Input: part model. Units: mm. Frame: model coordinates. Round coordinates to 2 decimals unless told otherwise and drop trailing zeros. Loops run counter-clockwise (first coordinate to the right, second up) from the corner with the lowest first, then second, coordinate; pieces in that order, holes last. Notation, with made-up numbers: (88, 72.5) -> (95, 72.5) arc R11 ccw to (95, 78.5) -> close; hole circle Ø8 at (60, 77). An arc over 180 degrees is marked (long way). Answer in a Markdown table with one row per item. Add a question column.
Q1. Pin query (flat end, axial travel): pin 1 (8 mm diameter, centred on y = 10.5, z = 4, fed in from +X); pin 2 (2 mm diameter, centred on y = -8.5, z = -0.5, fed in from -X). Return the tip coordinate at first contact, or that it passes through.
Q2. Section A-A, the plane z = -4.5. Output: boundary loops of the cut face in (x, y), and give its area (3 significant figures).
Q3. Mould query, pull axis X, two halves, no side actions, for faces 1 (the face through (13.404, -0.033, -6.511)), 2 (the face through (-13.404, -0.033, 6.511)), 3 (the face through (6.63, 0.87, 0.09)). Classes: pulls with the +X half, pulls with the -X half, needs draft (parallel to the pull), parting line crosses it, or undercut.
Q4. Ray query, L1, parallel to Y at x = 0, z = 2; L2, parallel to X at y = 2.75, z = 1.5; L3, parallel to Y at x = -2.25, z = -0.75. Return the intervals inside material, ascending. Write a range as from..to.
Solid Edge part; units mm, degrees
sketch "Sketch1" plane through (0, 0, 0) normal (0, 0, 1) x (1, 0, 0)
  line L0 (-7.5, -12.9904) -> (7.5, -12.9904)
  line L1 (7.5, -12.9904) -> (15, 0)
  line L2 (15, 0) -> (7.5, 12.9904)
  line L3 (7.5, 12.9904) -> (-7.5, 12.9904)
  line L4 (-7.5, 12.9904) -> (-15, 0)
  line L5 (-15, 0) -> (-7.5, -12.9904)
extrude "Protrusion1" add sketch "Sketch1" along normal mid plane 13.5
sketch "Sketch2" plane through (0, 0, 0) normal (1, 0, 0) x (0, 1, 0)
  line L0 (12.9904, -6.75) -> (34.5982, 5.7253)
revolve "RevolvedCutout1" cut sketch "Sketch2" angle 360 about axis through (0, 0, -57) along (0, 0, 1) material side at (0, 23.8193, -0.5557)
mirror "Mirror1" about plane through (0, 0, 0) normal (0, 0, 1) of "RevolvedCutout1"
hole "Hole_1" at (0, 0, 6.75) direction (0, 0, -1) diameter 13.376 end through all
properties part number "5" material "Fe - 410 W"
Answer block:
| question | item | result |
|---|---|---|
| 1 | pin 1 | x = 11.25 |
| 1 | pin 2 | x = -10.67 |
| 2 | outline | (-15, 0) -> (-7.5, -12.99) -> (7.5, -12.99) -> (15, 0) -> (7.5, 12.99) -> (-7.5, 12.99) -> close; hole circle Ø13.38 at (0, 0) |
| 2 | area | 444 mm^2 |
| 3 | face 1 | pulls with the +X half |
| 3 | face 2 | pulls with the -X half |
| 3 | face 3 | undercut |
| 4 | L1 | -12.99..-6.69, 6.69..12.99 |
| 4 | L2 | -13.41..-6.1, 6.1..13.41 |
| 4 | L3 | -12.99..-6.3, 6.3..12.99 |
